Can you work these out from the model? Positions are in its coordinate system, mm. Face numbers are marked on the shaded views. A direction names the side the tool comes from. Give positions to 0.01 mm unless a question says otherwise; leave off trailing zeros. Write each loop counter-clockwise with the first axis right and the second up, starting at its lowest first coordinate (ties: lowest second). Pieces come first, ordered by that corner, then holes.
1. Suppose I cut it at B-B (y = 11). Please give me the cut outline in (x, z), and give its area (3 significant figures).
2. If I drill on probe 1 along Z at (x, y) = (24.75, 29.7); probe 2 along Z at (x, y) = (24, 29); probe 3 along X at (y, z) = (23.5, -1.25), over which ranges is the centre line in solid material (lowest first)?
3. Suppose I cut it at A-A (x = 9). Please give me the cut outline in (y, z), and give its area (3 significant figures).
4. Suppose I cut it at C-C (z = 0). Please give me the cut outline in (x, y), and give its area (3 significant figures).
5. I'm going to push flat-ended pins straight in: pin 1 (3 mm diameter, centred on y = 34, z = 1.5, fed in from +X); pin 2 (12 mm diameter, centred on x = -5, z = 2, fed in from -Y); pin 3 (4.5 mm diameter, centred on x = 24.75, z = -5, fed in from +Y); pin 4 (2 mm diameter, centred on x = 16.5, z = 0, fed in from +Y). Where does each tip first touch, or does it pass through?
6. Suppose I cut it at D-D (x = 23). Please give me the cut outline in (y, z), and give its area (3 significant figures).
7. On a 3-axis mill with a long thin cutter (end or side, diameter ignored), from which of +Z, -Z, +X, -X, +Y, -Y can I reach the whole of each face in a straight line? I mean the marked faces 1, 2 and 3. Say none if no direction works.
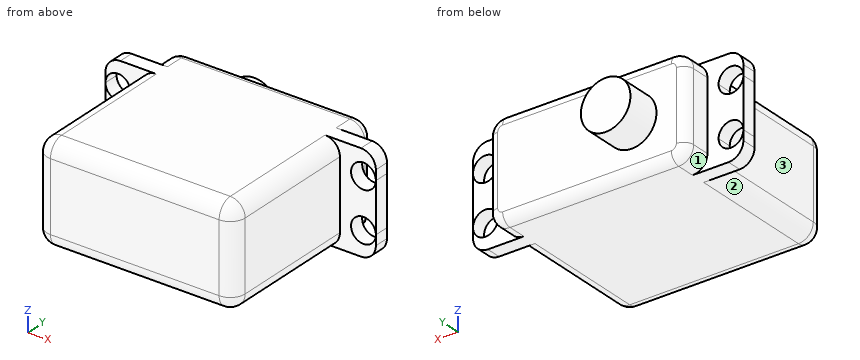
Autodesk Inventor part; units mm, degrees
ref_plane "YZ Plane" through (0, 0, 0) normal (1, 0, 0) x (0, 1, 0)
ref_plane "XZ Plane" through (0, 0, 0) normal (0, 1, 0) x (-1, 0, 0)
ref_plane "XY Plane" through (0, 0, 0) normal (0, 0, 1) x (1, 0, 0)
sketch "Boceto1" plane through (0, 0, 0) normal (0, 1, 0) x (-1, 0, 0)
  line L0 (20, 10) -> (-20, 10)
  line L1 (-20, 10) -> (-20, -10)
  line L2 (-20, -10) -> (20, -10)
  line L3 (20, -10) -> (20, 10)
  point P0 (0, 0)
  point P1 (-20, 0)
  dimension "d0" = 20
  dimension "d1" = 40
  dimension "d2" = 10
  dimension "d3" = 20
extrude "Extrusión1" add sketch "Boceto1" along normal blind 28.5
fillet "Empalme1" radius 3 4 edges at (0, 0, 10) (20, 0, 0) (0, 0, -10) (-20, 0, 0)
fillet "Empalme2" radius 3 6 edges at (-20, 15.75, -10) (-19.1213, 0.8787, -9.1213) (-20, 15.75, 10) (-19.1213, 0.8787, 9.1213) (20, 15.75, 10) (19.1213, 0.8787, 9.1213)
fillet "Empalme3" radius 3 2 edges at (20, 15.75, -10) (19.1213, 0.8787, -9.1213)
sketch "Boceto2" plane through (0, 28.5, 0) normal (0, 1, 0) x (1, 0, 0)
  line L0 (-27.25, 10) -> (27.25, 10)
  line L1 (27.25, 10) -> (27.25, -10)
  line L2 (27.25, -10) -> (-27.25, -10)
  line L3 (-27.25, -10) -> (-27.25, 10)
  line L4 (17, 10) -> (-17, 10)
  line L5 (-17, -10) -> (17, -10)
  point P0 (0, 0)
  dimension "d9" = 0
  dimension "d10" = 0
  dimension "d11" = 54.5
  dimension "d12" = 27.25
extrude "Extrusión2" add sketch "Boceto2" along normal blind 3
fillet "Empalme4" radius 3 3 edges at (-27.25, 30, 10) (-27.25, 30, -10) (27.25, 30, 10)
fillet "Empalme5" radius 3 1 edges at (27.25, 30, -10)
sketch "Boceto3" plane through (0, 31.5, 0) normal (0, 1, 0) x (1, 0, 0)
  line L0 (-17, 10) -> (17, 10)
  line L1 (-24.25, -10) -> (24.25, -10)
  line L2 (-20, 10) -> (20, 10)
  line L3 (20, 10) -> (20, -10)
  line L4 (20, -10) -> (-20, -10)
  line L5 (-20, -10) -> (-20, 10)
  point P0 (0, 0)
  dimension "d17" = 20
  dimension "d18" = 20
extrude "Extrusión3" add sketch "Boceto3" along normal blind 5.7
fillet "Empalme6" radius 3 3 edges at (20, 34.35, -10) (20, 34.35, 10) (-20, 34.35, -10)
fillet "Empalme7" radius 2 7 edges at (-20, 37.2, 1.5) (-19.1213, 37.2, -9.1213) (0, 37.2, -10) (19.1213, 37.2, -9.1213) (20, 37.2, 0) (19.1213, 37.2, 9.1213) (-1.5, 37.2, 10)
fillet "Empalme8" radius 3 2 edges at (-20, 33.35, 10) (-19.4142, 36.6142, 9.4142)
sketch "Boceto4" plane through (0, 31.5, 0) normal (0, 1, 0) x (1, 0, 0)
  circle A0 centre (-24.75, 5) radius 2.5
  line L0 (-38.2556, 0) -> (37.7734, 0)
  line L1 (0, 20.4997) -> (0, -23.7455)
  circle A1 centre (-24.75, -5) radius 2.5
  circle A2 centre (24.75, 5) radius 2.5
  circle A3 centre (24.75, -5) radius 2.5
  point P0 (0, 0)
  dimension "d24" = 24.75
  dimension "d25" = 5
  dimension "d26" = 5
  dimension "d27" = 24.75
extrude "Extrusión4" cut sketch "Boceto4" against normal blind 5
sketch "Boceto5" plane through (0, 37.2, 0) normal (0, 1, 0) x (1, 0, 0)
  circle A0 centre (-9, 0) radius 5
  point P0 (0, 0)
  dimension "d30" = 10
  dimension "d31" = 9
extrude "Extrusión5" add sketch "Boceto5" along normal blind 7
equation "\"Radio_pliegue\" = Grosor"
equation "\"Anchura_desahogo_plegado\" = Grosor"
equation "\"Profundidad_desahogo_plegado\" = 0.5 * Grosor"
equation "\"Tamaño_destalonado\" = 4 * Grosor"
equation "\"Remanente_mínimo\" = 2 * Grosor"
equation "\"Radiodetransición\" = Radio_pliegue"
equation "\"Tamaño_de_radio_de_Jacobi\" = Radio_pliegue"
equation "\"TamañoSeparación\" = Grosor"
properties part number "Feedback 360"
Checks:
1. outline: (-20, -7) arc R3 ccw to (-17, -10) - (17, -10) arc R3 ccw to (20, -7) - (20, 7) arc R3 ccw to (17, 10) - (-17, 10) arc R3 ccw to (-20, 7) - close
1. area: 792 mm2
2. probe 1: z = -9.96 to -7.5, -2.5 to 2.5, 7.5 to 9.96
2. probe 2: z = -10 to -7.38, -2.62 to 2.62, 7.38 to 10
2. probe 3: x = -20 to 20
3. outline: (0, -7) arc R3 ccw to (3, -10) - (35.2, -10) arc R2 ccw to (37.2, -8) - (37.2, 8) arc R2 ccw to (35.2, 10) - (3, 10) arc R3 ccw to (0, 7) - close
3. area: 738 mm2
4. outline: (-27.25, 28.5) - (-20, 28.5) - (-20, 3) arc R3 ccw to (-17, 0) - (17, 0) arc R3 ccw to (20, 3) - (20, 28.5) - (27.25, 28.5) - (27.25, 31.5) - (20, 31.5) - (20, 35.2) arc R2 ccw to (18, 37.2) - (-4, 37.2) - (-4, 44.2) - (-14, 44.2) - (-14, 37.2) - (-18, 37.2) arc R2 ccw to (-20, 35.2) - (-20, 31.5) - (-27.25, 31.5) - close
4. area: 1,600 mm2
5. pin 1: stops at x = 20
5. pin 2: stops at y = 0
5. pin 3: passes through
5. pin 4: stops at y = 37.2
6. outline: (28.5, -10) - (31.5, -10) - (31.5, -6.79) - (28.5, -6.79) - close; (28.5, -3.21) - (31.5, -3.21) - (31.5, 3.21) - (28.5, 3.21) - close; (28.5, 6.79) - (31.5, 6.79) - (31.5, 10) - (28.5, 10) - close
6. area: 38.6 mm2
7. face 1: -Z, -X, +Y
7. face 2: -Z, -X, -Y
7. face 3: +Z, -Z, -X, -Y
